```python
from build123d import *

# Parameters (mm, degrees)
SKETCH1_R           = 12.5
BOSS_EXTRUDE1_DEPTH = 93.6
SKETCH2_R           = 15
BOSS_EXTRUDE2_DEPTH = 56
SKETCH3_R           = 5.565
BOSS_EXTRUDE3_DEPTH = 45
SKETCH4_R           = 4.755
CUT_EXTRUDE1_DEPTH  = 60
FILLET2_R           = 2
FILLET3_R           = 1.5
FILLET4_R           = 2


with BuildPart() as part:
    # Sketch1 → Boss-Extrude1 (new body)
    with BuildSketch(Plane.XY):
        Circle(SKETCH1_R)
    extrude(amount=BOSS_EXTRUDE1_DEPTH)

    # Sketch2 → Boss-Extrude2 (add)
    with BuildSketch(Plane.XY.offset(76)):
        Circle(SKETCH2_R)
    extrude(amount=-BOSS_EXTRUDE2_DEPTH)

    # Sketch3 → Boss-Extrude3 (add)
    with BuildSketch(Plane(origin=(0, 0, 0), x_dir=(-1, 0, 0), z_dir=(0, 0, -1))):
        Circle(SKETCH3_R)
    extrude(amount=BOSS_EXTRUDE3_DEPTH)

    # Sketch4 → Cut-Extrude1 (cut)
    with BuildSketch(Plane.XY.offset(93.6)):
        Circle(SKETCH4_R)
    extrude(amount=-CUT_EXTRUDE1_DEPTH, mode=Mode.SUBTRACT)

    # Fillet2
    fillet2_edges = [part.edges().sort_by_distance(p)[0] for p in [
        (-12.5, 0, 76),
    ]]
    fillet(fillet2_edges, radius=FILLET2_R)

    # Fillet3
    fillet3_edges = [part.edges().sort_by_distance(p)[0] for p in [
        (-12.5, 0, 20),
    ]]
    fillet(fillet3_edges, radius=FILLET3_R)

    # Fillet4
    fillet4_edges = [part.edges().sort_by_distance(p)[0] for p in [
        (5.565, 0, 0),
    ]]
    fillet(fillet4_edges, radius=FILLET4_R)


solid = part.part
```
Work out the finished part from the listing and answer in its coordinate system (mm). A direction names the side the tool comes from. Round coordinates to 2 decimals unless told otherwise and drop trailing zeros. Write each loop counter-clockwise with the first axis right and the second up, starting at its lowest first coordinate (ties: lowest second). Pieces come first, ordered by that corner, then holes.
1) Determine the mould class of faces 1 (the face through (0, -5, 93.6)), 2 (the face through (4.535, 1.428, 64.02)), 3 (the face through (0, 0, 33.6)), 4 (the face through (11.923, 3.755, 85.691)) for opening direction Y: pulls with the +Y half, pulls with the -Y half, needs draft (parallel to the pull), parting line crosses it, or undercut.
2) Which of the six approach directions +Z, -Z, +X, -X, +Y, -Y give full straight-line access (tool end or side, diameter ignored) to faces 5 (the face through (-14.985, 0.66, 48.392)), 6 (the face through (0, -8, 0))?
3) A cutting plane is placed at D-D on z = -10. Determine the outline of the cut face in (x, y) (3 decimals), and give its area (3 significant figures).
4) Consider probe 1 along Y at (x, z) = (0, 62) (3 decimals); probe 2 along Z at (x, y) = (2, -1.25); probe 3 along Z at (x, y) = (6, -4.25). Determine where each line is inside the solid, lowest interval first.
5) Flat-ended cylindrical pins translate along their axes: P1, Ø1.5, axis at y = -1, z = -2, coming from the -X side; P2, Ø3, axis at x = -7.5, z = 34.5, coming from the +Y side; P3, Ø6, axis at x = 10.5, z = -20, coming from the -Y side; P4, Ø5, axis at x = 9.5, y = -7, coming from the -Z side. Find the tip coordinate at first contact, or state that the pin passes through.
6) A cutting plane is placed at A-A on y = 0. Determine the outline of the cut face in (x, z) (3 decimals).
7) A cutting plane is placed at C-C on z = 41. Determine the outline of the cut face in (x, y) (3 decimals), and give its area (3 significant figures).
Entries:
1. face 1: needs draft
1. face 2: undercut
1. face 3: undercut
1. face 4: parting line crosses it
2. face 5: +Z, -Z
2. face 6: -Z
3. outline: circle Ø11.13 at (0, 0)
3. area: 97.3 mm2
4. probe 1: y = -15 to -4.755, 4.755 to 15
4. probe 2: z = -45 to 33.6
4. probe 3: z = -0.01 to 93.6
5. P1: stops at x = -5.64
5. P2: stops at y = 13.75
5. P3: passes through
5. P4: stops at z = 0
6. outline: (-15, 20) - (-14, 20) arc R1.5 cw to (-12.5, 18.5) - (-12.5, 0) - (-7.565, 0) arc R2 cw to (-5.565, -2) - (-5.565, -45) - (5.565, -45) - (5.565, -2) arc R2 cw to (7.565, 0) - (12.5, 0) - (12.5, 18.5) arc R1.5 cw to (14, 20) - (15, 20) - (15, 76) - (14.5, 76) arc R2 cw to (12.5, 78) - (12.5, 93.6) - (4.755, 93.6) - (4.755, 33.6) - (-4.755, 33.6) - (-4.755, 93.6) - (-12.5, 93.6) - (-12.5, 78) arc R2 cw to (-14.5, 76) - (-15, 76) - close
7. outline: circle Ø30 at (0, 0); hole circle Ø9.51 at (0, 0)
7. area: 636 mm2
